Verification items for this drawing (mm, ordinates from the low corner). Coordinates: 2 decimals unless noted, no trailing zeros. Loops run counter-clockwise (first coordinate to the right, second up) from the corner with the lowest first, then second, coordinate; pieces in that order, holes last. Notation, with made-up numbers: (-20, 67.25) - (-5, 67.25) arc R12 ccw to (-5, 87.25) - close; hole circle Ø10 at (79, 49.5). An arc over 180 degrees is marked (long way). One line per item, written item: value. Start each with the question number.
(1) Thickness scan on probe 1 along Y at (x, z) = (4.95, 3.1); probe 2 along X at (y, z) = (5, 3.95); probe 3 along Y at (x, z) = (3, 1.2). Record the ranges inside material, lowest first. Write a range as [from, to].
(2) Section check A-A (y = 5). Record the boundary of the cut face in (x, z).
(3) Section check B-B (x = 4.95). Record the boundary of the cut face in (y, z).
(4) Section check C-C (z = 2.2). Record the boundary of the cut face in (x, y), plus the area to 3 significant figures.
(5) Draft check along Y on the marked faces 1, 2 and 3. Enter one of: +Y half, -Y half, draft (parallel to the pull), parting line (faces both ways), or undercut.
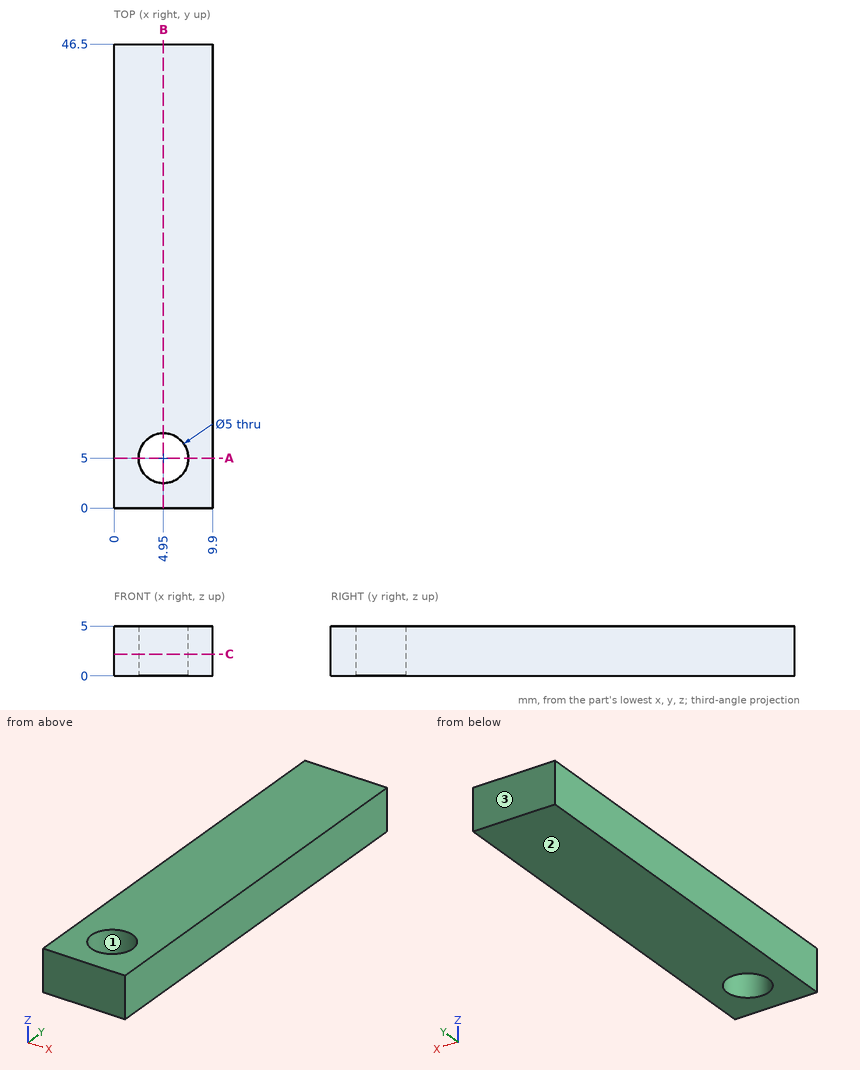
Responses:
1. probe 1: y = [0, 2.5], [7.5, 46.5]
1. probe 2: x = [0, 2.45], [7.45, 9.9]
1. probe 3: y = [0, 3.44], [6.56, 46.5]
2. outline: (0, 0) - (2.45, 0) - (2.45, 5) - (0, 5) - close; (7.45, 0) - (9.9, 0) - (9.9, 5) - (7.45, 5) - close
3. outline: (0, 0) - (2.5, 0) - (2.5, 5) - (0, 5) - close; (7.5, 0) - (46.5, 0) - (46.5, 5) - (7.5, 5) - close
4. outline: (0, 0) - (9.9, 0) - (9.9, 46.5) - (0, 46.5) - close; hole circle Ø5 at (4.95, 5)
4. area: 441 mm²
5. face 1: undercut
5. face 2: draft
5. face 3: +Y half
